The model under review builds one solid part; all positions refer to its coordinate system, in mm. Face numbers are marked on the shaded views. A direction names the side the tool comes from. Round coordinates to 2 decimals unless told otherwise and drop trailing zeros. Order: outer loops, then holes, each group sorted by start corner. A loop starts at its lowest first (then second) coordinate and runs counter-clockwise, first axis right, second up. Notation, with made-up numbers: M 27,78 L 64,78 A19 ccw 64,98 Z; hole C 63.25,-25 d6. An arc over 180 degrees is marked long. Use a Markdown table: item, result. Add a question column.
1. The part is to be moulded in two halves that separate along Y. For the marked faces 1, 2 and 3, say which applies: +Y half, -Y half, draft (parallel to the pull), parting line (faces both ways), or undercut.
2. For the marked faces 4, 5 and 6, list the 3-axis set-ups (+Z, -Z, +X, -X, +Y, -Y) from which the entire face can be reached by the end or side of a thin tool; tool diameter is ignored.
3. To check wall thickness, follow probe 1 along Y at (x, z) = (0, 11.5); probe 2 along X at (y, z) = (22, 11); probe 3 along Z at (x, y) = (21.5, 30). State the ranges of each line that lie inside material, in increasing order.
4. Insertion check: P1, Ø2, axis at x = -40, z = 54, coming from the +Y side; P2, Ø5, axis at x = 7, z = 13.5, coming from the +Y side; P3, Ø10, axis at x = 34, z = 5.5, coming from the +Y side. Each pin has a flat end and moves straight along its axis. Give the tip position at first contact, or say it passes through.
5. Consider section B-B on y = 4. State the section outline as (x, z) points.
6. Consider section A-A on x = 0. State the section outline as (y, z) points, then the cut area to 3 significant figures.
7. Consider section D-D on z = 71.5. State the section outline as (x, y) points, then the cut area to 3 significant figures.
8. Consider section C-C on x = -29. State the section outline as (y, z) points, then the cut area to 3 significant figures.
from build123d import *

# Parameters (mm, degrees)
SKETCH1_R           = 20
BOSS_EXTRUDE1_DEPTH = 20
SKETCH2_W           = 100
SKETCH2_H           = 20
BOSS_EXTRUDE2_DEPTH = 60


with BuildPart() as part:
    # Sketch1 → Boss-Extrude1 (new body)
    with BuildSketch(Plane.XY):
        with BuildLine():
            Line((-50, 22.5), (-25, 22.5))
            ThreePointArc((-25, 22.5), (0, 47.5), (25, 22.5))
            Line((25, 22.5), (50, 22.5))
            Line((50, 22.5), (50, -22.5))
            Line((50, -22.5), (-50, -22.5))
            Line((-50, -22.5), (-50, 22.5))
        make_face()
        with Locations((0, 22.5)):
            Circle(SKETCH1_R, mode=Mode.SUBTRACT)
    extrude(amount=BOSS_EXTRUDE1_DEPTH)

    # Sketch2 → Boss-Extrude2 (add)
    with BuildSketch(Plane.XY.offset(20)):
        with Locations((0, -12.5)):
            Rectangle(SKETCH2_W, SKETCH2_H)
    extrude(amount=BOSS_EXTRUDE2_DEPTH)


solid = part.part
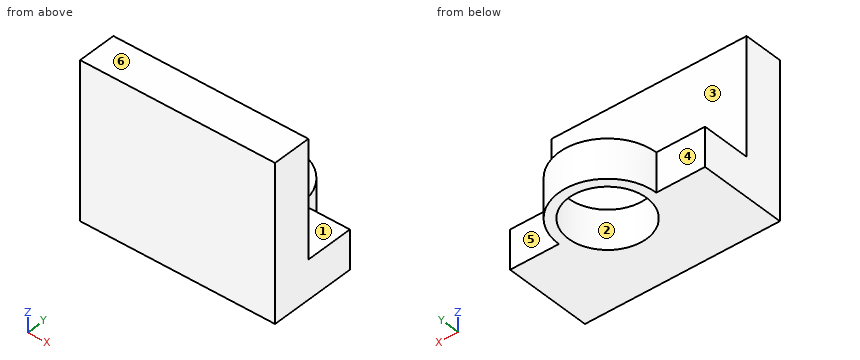
Answer block:
| question | item | result |
|---|---|---|
| 1 | face 1 | draft |
| 1 | face 2 | undercut |
| 1 | face 3 | +Y half |
| 2 | face 4 | +Z, -Z, -X, +Y |
| 2 | face 5 | +Z, -Z, +X, +Y |
| 2 | face 6 | +Z, +X, -X, +Y, -Y |
| 3 | probe 1 | -22.5 to 2.5, 42.5 to 47.5 |
| 3 | probe 2 | -50 to -19.99, 19.99 to 50 |
| 3 | probe 3 | 0 to 20 |
| 4 | P1 | y = -2.5 |
| 4 | P2 | y = 47.09 |
| 4 | P3 | y = 22.5 |
| 5 | outline | M -50,0 L -7.6,0 L -7.6,20 L -50,20 Z; M 7.6,0 L 50,0 L 50,20 L 7.6,20 Z |
| 6 | outline | M -22.5,0 L 2.5,0 L 2.5,20 L -2.5,20 L -2.5,80 L -22.5,80 Z; M 42.5,0 L 47.5,0 L 47.5,20 L 42.5,20 Z |
| 6 | area | 1,800 mm^2 |
| 7 | outline | M -50,-22.5 L 50,-22.5 L 50,-2.5 L -50,-2.5 Z |
| 7 | area | 2,000 mm^2 |
| 8 | outline | M -22.5,0 L 22.5,0 L 22.5,20 L -2.5,20 L -2.5,80 L -22.5,80 Z |
| 8 | area | 2,100 mm^2 |
